```python
from build123d import *

# Parameters (mm, degrees)
BOSS_EXTRUDE2_DEPTH = 15.38
BOSS_EXTRUDE3_DEPTH = 1
BOSS_EXTRUDE4_DEPTH = 12.38
CUT_EXTRUDE1_DEPTH  = 8.26
SKETCH12_R          = 4
CUT_EXTRUDE2_DEPTH  = 8.26
CUT_EXTRUDE3_DEPTH  = 3
SKETCH16_W          = 10
SKETCH16_H          = 2
CUT_EXTRUDE4_DEPTH  = 3
CUT_EXTRUDE5_DEPTH  = 13
CUT_EXTRUDE6_DEPTH  = 1


with BuildPart() as part:
    # Sketch1 → Boss-Extrude2 (new body)
    with BuildSketch(Plane(origin=(0, 0, 0), x_dir=(1, 0, 0), z_dir=(0, 1, 0))):
        Polygon((-33.232050802, 130.626242439), (-11.732050802, 167.865334802), (3.267949197, 159.205080764), (-18.232050803, 121.965988402), (-18.732050803, 121.099962998), (-16.133974592, 119.599962998), (13.464101619, 170.865334801), (2.556624332, 189.757639644), (-2.556624322, 189.757639644), (-112.11324865, 2e-09), (-109.556624323, -4.428203228), (-87.74166975, -4.428203228), (-62.14359354, 39.908965344), (-64.74166975, 41.408965344), (-65.74166975, 39.676914536), (-82.74166975, 10.232050807), (-87.74166975, 1.57179677), (-97.741669749, 18.892304845), (-80.741669749, 48.337168573), (-79.741669749, 50.069219381), (-33.732050802, 129.760217035), align=None)
        Polygon((-89.473720558, -1.42820323), (-107.824573519, -1.42820323), (-108.649147039, 0), (-99.473720558, 15.892304845), align=None, mode=Mode.SUBTRACT)
        Polygon((-9.999999996, 170.865334801), (-0.824573515, 186.757639646), (0.824573508, 186.757639646), (10.000000004, 170.865334801), align=None, mode=Mode.SUBTRACT)
    extrude(amount=BOSS_EXTRUDE2_DEPTH)

    # Sketch1_11 → Boss-Extrude3 (add)
    with BuildSketch(Plane(origin=(0, 0, 0), x_dir=(1, 0, 0), z_dir=(0, 1, 0))):
        Polygon((3.267949197, 159.205080764), (-11.732050802, 167.865334802), (-33.232050802, 130.626242439), (-18.232050803, 121.965988402), align=None)
        Polygon((-65.74166975, 39.676914536), (-80.741669749, 48.337168573), (-97.741669749, 18.892304845), (-87.74166975, 1.57179677), align=None)
    extrude(amount=BOSS_EXTRUDE3_DEPTH)

    # Sketch1_12 → Boss-Extrude4 (add)
    with BuildSketch(Plane(origin=(0, 0, 0), x_dir=(1, 0, 0), z_dir=(0, 1, 0))):
        Polygon((-33.732050802, 129.760217035), (-33.232050802, 130.626242439), (-18.232050803, 121.965988402), (-18.732050803, 121.099962998), align=None)
        Polygon((-64.74166975, 41.408965344), (-79.741669749, 50.069219381), (-80.741669749, 48.337168573), (-65.74166975, 39.676914536), align=None)
    extrude(amount=BOSS_EXTRUDE4_DEPTH)

    # Sketch10 → Cut-Extrude1 (cut)
    with BuildSketch(Plane(origin=(47.754809476, 0, -82.713756318), x_dir=(0.8660254037844418, 0, 0.49999999999999456), z_dir=(-0.4999999999999946, 0, 0.8660254037844419))):
        Polygon((-85.432921433, 5), (-81.432921433, 5), (-81.432921433, 9), (-89.432921433, 9), (-89.432921433, 5), align=None)
    extrude(amount=-CUT_EXTRUDE1_DEPTH, mode=Mode.SUBTRACT)

    # Sketch12 → Cut-Extrude2 (cut)
    with BuildSketch(Plane(origin=(1.745190528, 0, -3.022758664), x_dir=(-0.866025403784436, 0, -0.5000000000000047), z_dir=(0.5000000000000047, 0, -0.866025403784436))):
        with Locations((85.432921433, 6.5)):
            Circle(SKETCH12_R)
    extrude(amount=-CUT_EXTRUDE2_DEPTH, mode=Mode.SUBTRACT)

    # Sketch15 → Cut-Extrude3 (cut)
    with BuildSketch(Plane.XZ):
        Polygon((-87.74166975, 4.428203228), (-109.556624323, 4.428203228), (-112.11324865, -2e-09), (-101.205771363, -18.892304845), align=None)
        Polygon((13.464101619, -170.865334801), (2.556624332, -189.757639644), (-2.556624322, -189.757639644), (-13.464101609, -170.865334801), align=None)
    extrude(amount=-CUT_EXTRUDE3_DEPTH, mode=Mode.SUBTRACT)

    # Sketch16 → Cut-Extrude4 (cut)
    with BuildSketch(Plane(origin=(-84.084936489, 0, -48.546460716), x_dir=(-0.4999999999999999, 0, 0.8660254037844386), z_dir=(-0.8660254037844387, 0, -0.49999999999999994))):
        with Locations((-133.242624333, 2)):
            Rectangle(SKETCH16_W, SKETCH16_H)
        with Locations((26.242624323, 2)):
            Rectangle(SKETCH16_W, SKETCH16_H)
    extrude(amount=-CUT_EXTRUDE4_DEPTH, mode=Mode.SUBTRACT)

    # Sketch17 → Cut-Extrude5 (cut)
    with BuildSketch(Plane(origin=(0, 15.38, 0), x_dir=(1, 0, 0), z_dir=(0, 1, 0))):
        Polygon((-18.232050803, 121.965988402), (-17.366025399, 121.465988402), (4.633974601, 159.571106168), (-12.098076205, 169.231360205), (-34.098076205, 131.126242439), (-33.232050802, 130.626242439), align=None)
    extrude(amount=-CUT_EXTRUDE5_DEPTH, mode=Mode.SUBTRACT)

    # Sketch18 → Cut-Extrude6 (cut)
    with BuildSketch(Plane.XZ):
        Polygon((-18.232050803, -121.965988402), (3.267949197, -159.205080764), (-11.732050802, -167.865334802), (-33.232050802, -130.626242439), align=None)
    extrude(amount=-CUT_EXTRUDE6_DEPTH, mode=Mode.SUBTRACT)


solid = part.part
```
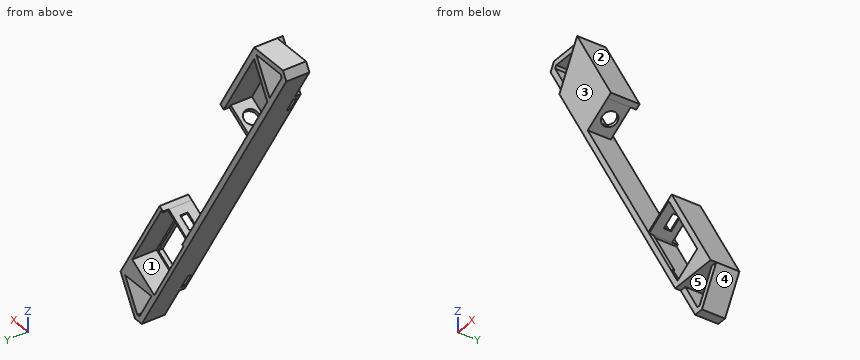
The listing builds one solid part. Answer for the finished solid, in the listing's coordinates (mm). Face numbers are marked on the shaded views. A direction names the side the tool comes from. Round coordinates to 2 decimals unless told otherwise and drop trailing zeros. Loops run counter-clockwise (first coordinate to the right, second up) from the corner with the lowest first, then second, coordinate; pieces in that order, holes last.
Q1. Section D-D, the plane x = -73 is taken. Count the separate pieces of the cut face and the enclosed holes in it, then the cut area to 3 significant figures.
Q2. Find the intervals of material crossed by line 1 (Z direction, x = -5, y = 10.75); line 2 (Z direction, x = 2.5, y = 14); line 3 (Z direction, x = -81, y = 1.75), in increasing order.
Q3. Given pin 1 Ø5.5 at (x, z) = (3.5, -184) entering from -Y; pin 2 Ø8 at (y, z) = (7, -19) entering from +X; pin 3 Ø0.8 at (x, y) = (0, 9.5) entering from +Z, each flat-ended and moving along its own axis, determine where each tip first touches the part or whether it passes through.
Q4. Section A-A, the plane z = -141.5 is taken. Determine the outline of the cut face in (x, y).
Q5. Section B-B, the plane x = -6 is taken. Determine the outline of the cut face in (y, z), then the cut area to 3 significant figures.
Q6. For a pull along Z with two mould halves and no side action, classify the marked faces 3, 4 and 5 as released by +Z, released by -Z, zero draft, split by the parting line, or undercut.
Q7. Which of the six approach directions +Z, -Z, +X, -X, +Y, -Y give full straight-line access (tool end or side, diameter ignored) to the marked faces 1 and 2?
Q8. Section C-C, the plane z = -91 is taken. Determine the outline of the cut face in (x, y), then the cut area to 3 significant figures.
Completed:
1. separate pieces: 3
1. enclosed holes: 0
1. area: 212 mm2
2. line 1: z = -185.53 to -179.53, -170.87 to -165.13, -142.88 to -138.88
2. line 2: z = -189.76 to -183.86, -170.87 to -160.8, -155.87 to -151.87
2. line 3: z = -53.89 to -47.89, -13.25 to -7.25
3. pin 1: stops at y = 3
3. pin 2: stops at x = -71.91
3. pin 3: stops at z = -146.85
4. outline: (-30.42, 0) - (-26.95, 0) - (-26.95, 2.38) - (-28.11, 2.38) - (-28.11, 15.38) - (-30.42, 15.38) - close; (-6.95, 0) - (-3.49, 0) - (-3.49, 15.38) - (-5.8, 15.38) - (-5.8, 2.38) - (-6.95, 2.38) - close
5. outline: (0, -170.87) - (15.38, -170.87) - (15.38, -165.71) - (2.38, -165.71) - (2.38, -164.56) - (0, -164.56) - close; (0, -143.15) - (2.38, -143.15) - (2.38, -141.15) - (15.38, -141.15) - (15.38, -137.15) - (0, -137.15) - close; (3, -183.79) - (15.38, -183.79) - (15.38, -177.79) - (3, -177.79) - close
5. area: 223 mm2
6. face 3: zero draft
6. face 4: released by -Z
6. face 5: undercut
7. face 1: +Y
7. face 2: +Z, +X, +Y, -Y
8. outline: (-59.57, 0) - (-56.11, 0) - (-56.11, 15.38) - (-59.57, 15.38) - close
8. area: 53.3 mm2
